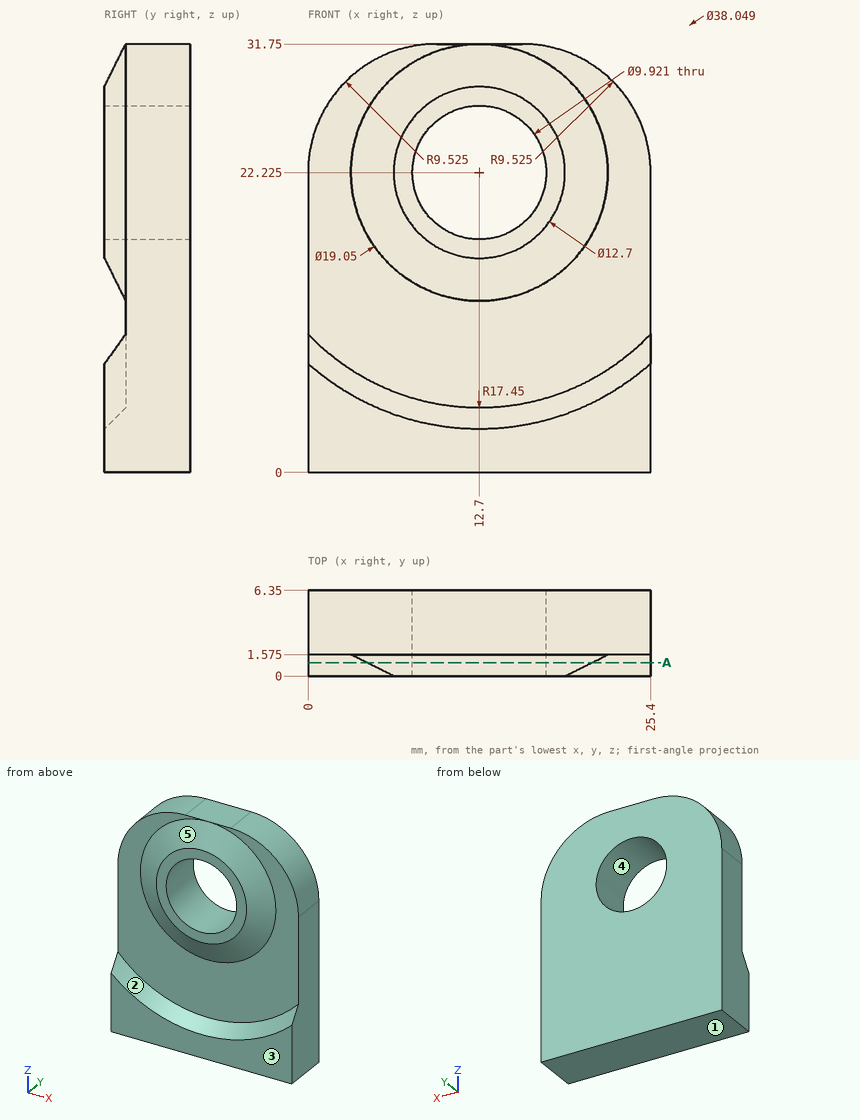
Part print with two shaded views. Sizes in mm from the minimum x, y, z corner. A direction names the side the tool comes from. Coordinates: 2 decimals unless noted, no trailing zeros. Write each loop counter-clockwise with the first axis right and the second up, starting at its lowest first coordinate (ties: lowest second). Pieces come first, ordered by that corner, then holes.
(1) 3-axis set-ups, long thin cutter, end or side, ignore diameter. For the marked faces 1 and 2: which of +Z, -Z, +X, -X, +Y, -Y reach the whole face in a straight line?
(2) Mould opens along X. For the marked faces 3, 4 and 5 say: pulls with the +X half, pulls with the -X half, needs draft (parallel to the pull), parting line crosses it, or undercut.
(3) Cut at A-A on y = 1. List the corners of the cut face in (x, z) (1 decimal), and give its area (3 significant figures).
(4) Drill centre lines: line 1 (Z direction, x = 12.7, y = 2.5); line 2 (Z direction, x = 16, y = 1.25); line 3 (X direction, y = 1.5, z = 23). Where is each one in solid material? Low to high.
(5) Pin check, flat tips, straight feed: pin 1 Ø3 at (x, y) = (22, 5) entering from +Z; pin 2 Ø2 at (x, z) = (11.5, 7) entering from -Y (3 decimals). Stop position of each tip, or through.
Working result:
1. face 1: -Z, +X, -X, +Y, -Y
1. face 2: -Y
2. face 3: needs draft
2. face 4: undercut
2. face 5: parting line crosses it
3. outline: (0, 0) - (25.4, 0) - (25.4, 9.4) arc R18 cw to (0, 9.4) - close; circle Ø16.7 at (12.7, 22.2); hole circle Ø9.9 at (12.7, 22.2)
3. area: 291 mm2
4. line 1: z = 0 to 17.26, 27.19 to 31.75
4. line 2: z = 0 to 4.76, 13.99 to 18.52, 25.93 to 30.46
4. line 3: x = 3.36 to 7.8, 17.6 to 22.04
5. pin 1: stops at z = 30.55
5. pin 2: stops at y = 1.575
